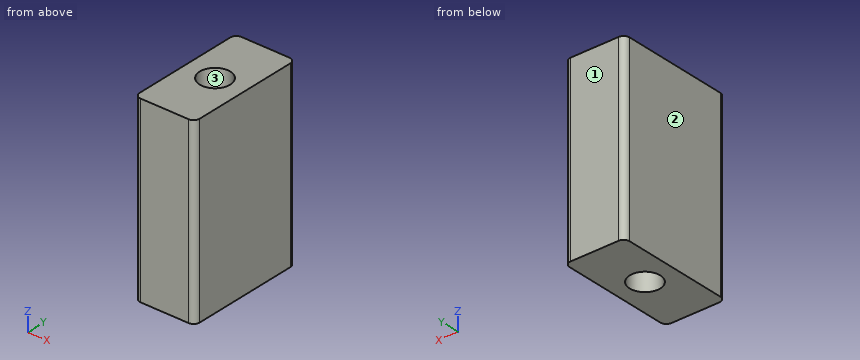
```python
from build123d import *

# Parameters (mm, degrees)
F0_W     = 50.8
F0_H     = 101.6
F0_R     = 12.923254
F1_DEPTH = 153.924
F2_R     = 5.08


with BuildPart() as f1:
    # F0 (on Top) → F1 (new body)
    with BuildSketch(Plane.XY):
        with Locations((25.4, 50.8)):
            Rectangle(F0_W, F0_H)
        with Locations((25.4, 50.8)):
            Circle(F0_R, mode=Mode.SUBTRACT)
    extrude(amount=-F1_DEPTH)

    # F2
    f2_edges = [f1.edges().sort_by_distance(p)[0] for p in [
        (50.8, 0, -76.962),
        (50.8, 101.6, -76.962),
        (0, 0, -76.962),
        (0, 101.6, -76.962),
    ]]
    fillet(f2_edges, radius=F2_R)


solid = f1.part
```
Could you check a few things on this model? Use its own coordinates, in mm. Face numbers are marked on the shaded views. Give positions to 0.01 mm unless a question says otherwise; leave off trailing zeros. Write each loop counter-clockwise with the first axis right and the second up, starting at its lowest first coordinate (ties: lowest second). Pieces come first, ordered by that corner, then holes. Notation, with made-up numbers: (-36.5, 74) - (-26.5, 74) arc R20 cw to (-26.5, 81) - close; hole circle Ø3 at (47, 51.5). An arc over 180 degrees is marked (long way). One line per item, written item: value. Start each with the question number.
Item 1: Please list where these lines run through material, in increasing order: line 1 (Y direction, x = 25.4, z = -116); line 2 (X direction, y = 50, z = -33); line 3 (X direction, y = 44, z = -32). Write a range as from..to.
Item 2: I'm going to push a flat-ended pin straight in: pin 1 (6 mm diameter, centred on x = 13.5, y = 45.5, fed in from +Z). Where does the tip first touch, or does it pass through?
Item 3: Imagine slicing it at B-B, the plane z = -100. List the corners of the cut face in (x, y) for me, and give its area (3 significant figures).
Item 4: Imagine slicing it at C-C, the plane x = 25.4. List the corners of the cut face in (y, z) for me, and give its area (3 significant figures).
Item 5: Imagine slicing it at A-A, the plane y = 50.8. List the corners of the cut face in (x, z) for me.
Item 6: If we mould it in two halves opening along X, with no side actions, what happens to the marked faces 1, 2 and 3? For each: +X half, -X half, draft (parallel to the pull), parting line (faces both ways), or undercut.
Geometry says:
1. line 1: 0..37.88, 63.72..101.6
1. line 2: 0..12.5, 38.3..50.8
1. line 3: 0..14.41, 36.39..50.8
2. pin 1: z = 0
3. outline: (0, 5.08) arc R5.08 ccw to (5.08, 0) - (45.72, 0) arc R5.08 ccw to (50.8, 5.08) - (50.8, 96.52) arc R5.08 ccw to (45.72, 101.6) - (5.08, 101.6) arc R5.08 ccw to (0, 96.52) - close; hole circle Ø25.85 at (25.4, 50.8)
3. area: 4,610 mm^2
4. outline: (0, -153.92) - (37.88, -153.92) - (37.88, 0) - (0, 0) - close; (63.72, -153.92) - (101.6, -153.92) - (101.6, 0) - (63.72, 0) - close
4. area: 11,700 mm^2
5. outline: (0, -153.92) - (12.48, -153.92) - (12.48, 0) - (0, 0) - close; (38.32, -153.92) - (50.8, -153.92) - (50.8, 0) - (38.32, 0) - close
6. face 1: draft
6. face 2: -X half
6. face 3: undercut
